```python
from build123d import *

# Parameters (mm, degrees)
F0_R     = 6.35
F1_DEPTH = 11.176
F0_R_2   = 16.256
F0_R_3   = 14.2875
F2_DEPTH = 41.148
F3_R     = 3.048
F4_R     = 3.048


with BuildPart() as f1:
    # F0 (on Top) → F1 (new body)
    with BuildSketch(Plane.XY):
        with BuildLine():
            ThreePointArc((-41.3472187621, 3.175), (-41.1978536154, 1.5906219786), (-41.148, 0))
            ThreePointArc((-41.148, 0), (-41.1978536154, -1.5906219786), (-41.3472187621, -3.175))
            Line((-41.3472187621, -3.175), (0, -3.175))
            Line((0, -3.175), (0, 0))
            Line((0, 0), (0, 3.175))
            Line((0, 3.175), (-41.3472187621, 3.175))
        make_face()
        with BuildLine():
            Line((0, -3.175), (-41.3472187621, -3.175))
            ThreePointArc((-41.3472187621, -3.175), (-54.1727312933, -22.1813598419), (-77.0827467531, -23.1123151339))
            Line((-77.0827467531, -23.1123151339), (-23.6490600649, -47.4677444402))
            ThreePointArc((-23.6490600649, -47.4677444402), (-10.6164287508, -48.4793380387), (0, -40.8527895955))
            Line((0, -40.8527895955), (0, -3.175))
        make_face()
        with Locations((-15.748, -30.1335080897)):
            Circle(F0_R, mode=Mode.SUBTRACT)
    extrude(amount=F1_DEPTH)

    # F0 (on Top) → F2 (join)
    with BuildSketch(Plane.XY):
        with BuildLine():
            ThreePointArc((-41.3472187621, -3.175), (-41.1978536154, -1.5906219786), (-41.148, 0))
            ThreePointArc((-41.148, 0), (-41.1978536154, 1.5906219786), (-41.3472187621, 3.175))
            ThreePointArc((-41.3472187621, 3.175), (-53.9498972239, 22.0555618029), (-76.6149503625, 23.3198737218))
            ThreePointArc((-76.6149503625, 23.3198737218), (-91.9467110203, 0.2558876856), (-77.0827467531, -23.1123151339))
            ThreePointArc((-77.0827467531, -23.1123151339), (-54.1727312933, -22.1813598419), (-41.3472187621, -3.175))
        make_face()
        with Locations((-66.548, 0)):
            Circle(F0_R_2, mode=Mode.SUBTRACT)
        with Locations((-66.548, 0)):
            Circle(F0_R_2)
        with Locations((-66.548, 0)):
            Circle(F0_R_3, mode=Mode.SUBTRACT)
    extrude(amount=F2_DEPTH)

    # F3
    f3_edges = [f1.edges().sort_by_distance(p)[0] for p in [
        (-91.748781, 3.175, 41.148),
    ]]
    fillet(f3_edges, radius=F3_R)

    # F4
    f4_edges = [f1.edges().sort_by_distance(p)[0] for p in [
        (-80.8355, 0, 41.148),
    ]]
    fillet(f4_edges, radius=F4_R)


solid = f1.part
```
Verification items for the finished model (mm, model axes). A direction names the side the tool comes from. Round coordinates to 2 decimals unless told otherwise and drop trailing zeros. Write each loop counter-clockwise with the first axis right and the second up, starting at its lowest first coordinate (ties: lowest second). Pieces come first, ordered by that corner, then holes.
1. Access from +Z, -Z, +X, -X, +Y, -Y to the whole of each face (thin tool, end or side, straight path). Record for faces 1 (the cylindrical face through (-10.8, -48.53, 5.51)), 2 (the flat face through (-20, 3.175, 6)).
2. Gauge pin test, flat ends, axial feed: P1, Ø12, axis at x = -22, y = -0.5, coming from the +Z side; P2, Ø1.5, axis at x = -73.5, y = 11, coming from the -Z side; P3, Ø10, axis at x = -29.5, z = 7, coming from the +Y side (3 decimals); P4, Ø1, axis at y = 8.5, z = 9, coming from the -X side. Record the tip position at first contact, or that the pin passes through.
3. Section check A-A on x = -17. Enter the section's corners in (y, z) (3 decimals), plus the area to 3 significant figures.
4. Section check C-C on z = 9. State how many separate pieces and enclosed holes the cut face has, plus the area to 3 significant figures.
5. Draft check along Y on faces 3 (the cylindrical face through (-12.82, -35.77, 5.51)), 4 (the flat face through (-51, -35, 6)), 5 (the flat face through (-47, -11, 0)). Enter one of: +Y half, -Y half, draft (parallel to the pull), parting line (faces both ways), or undercut.
6. Scan lines: L1, parallel to X at y = -3.5, z = 26; L2, parallel to X at y = 9.5, z = 19; L3, parallel to Z at x = -43.5, y = -22.5. Record each from-to range of solid material in increasing order.
7. Section check B-B on z = 15. Enter the section's corners in (x, y) (1 decimal), plus the area to 3 significant figures.
8. Section check D-D on x = -29. Enter the section's corners in (y, z) (3 decimals), plus the area to 3 significant figures.
Answer:
1. face 1: +Z, -Z, -Y
1. face 2: +Z, -Z, +X, +Y
2. P1: stops at z = 11.18
2. P2: passes through
2. P3: stops at y = 3.175
2. P4: stops at x = -90.66
3. outline: (-49.142, 0) - (-36.359, 0) - (-36.359, 11.176) - (-49.142, 11.176) - close; (-23.908, 0) - (3.175, 0) - (3.175, 11.176) - (-23.908, 11.176) - close
3. area: 446 mm2
4. separate pieces: 1
4. enclosed holes: 2
4. area: 3,630 mm2
5. face 3: undercut
5. face 4: -Y half
5. face 5: draft
6. L1: x = -91.71 to -80.4, -52.7 to -41.39
6. L2: x = -90.1 to -77.22, -55.88 to -42.99
6. L3: z = 0 to 11.18
7. outline: circle Ø50.8 at (-66.5, 0); hole circle Ø28.6 at (-66.5, 0)
7. area: 1,390 mm2
8. outline: (-45.029, 0) - (3.175, 0) - (3.175, 11.176) - (-45.029, 11.176) - close
8. area: 539 mm2
